Input: part model. Units: mm. Frame: model coordinates. Face numbers are marked on the shaded views. A direction names the side the tool comes from. Round coordinates to 2 decimals unless told otherwise and drop trailing zeros. Loops run counter-clockwise (first coordinate to the right, second up) from the corner with the lowest first, then second, coordinate; pieces in that order, holes last.
(1) First-contact query: pin 1 Ø1 at (x, y) = (17.5, 2) entering from +Z. Flat tip, straight axial feed; report the tip coordinate or a pass-through.
(2) Line query: line 1 (X direction, y = 2, z = 1.25); line 2 (X direction, y = 2, z = 3.1); line 3 (Y direction, x = 2.5, z = 1.85). Output: solid intervals per line, ascending.
(3) Draft query along Y for the marked faces 1, 2 and 3. Return one class per face: released by +Y, released by -Y, zero draft, split by the parting line, or undercut.
(4) Cut plane B-B, the plane z = 1.25. Output: boundary loops of the cut face in (x, y), and give its area (3 significant figures).
(5) Cut plane D-D, the plane z = 3. Output: boundary loops of the cut face in (x, y), and give its area (3 significant figures).
(6) Cut plane A-A, the plane y = 2. Output: boundary loops of the cut face in (x, z).
(7) Cut plane C-C, the plane x = 2.5. Output: boundary loops of the cut face in (y, z), and give its area (3 significant figures).
(8) Access query for the marked faces 4 and 5. Directions: +Z, -Z, +X, -X, +Y, -Y. A direction counts if a zero-diameter tool reaches every point of the face in a straight line with its end or side. Return the directions, or none.
Autodesk Inventor part; units mm, degrees
ref_plane "YZ Plane" through (0, 0, 0) normal (1, 0, 0) x (0, 1, 0)
ref_plane "XZ Plane" through (0, 0, 0) normal (0, 1, 0) x (-1, 0, 0)
ref_plane "XY Plane" through (0, 0, 0) normal (0, 0, 1) x (1, 0, 0)
sketch "Sketch1" plane through (0, 0, 0) normal (0, 0, 1) x (1, 0, 0)
  line L0 (0, 0) -> (20, 0)
  line L1 (20, 0) -> (20, 4)
  line L2 (20, 4) -> (0, 4)
  line L3 (0, 4) -> (0, 0)
  dimension "d0" = 20
  dimension "d1" = 4
extrude "Extrusion1" add sketch "Sketch1" along normal blind 4
sketch "Sketch2" plane through (0, 0, 0) normal (0, -1, 0) x (1, 0, 0)
  line L0 (5.5, 0) -> (14.5, 0)
  line L1 (14.5, 0) -> (14.5, 2)
  line L2 (14.5, 2) -> (5.5, 2)
  line L3 (5.5, 2) -> (5.5, 0)
  line L4 (0, 0) -> (20, 0) construction
  line L5 (10, 0) -> (10, 4) construction
  line L6 (0, 4) -> (20, 4) construction
  dimension "d4" = 9
  dimension "d5" = 2
extrude "Extrusion2" cut sketch "Sketch2" against normal blind 4
sketch "Sketch3" plane through (0, 0, 4) normal (0, 0, 1) x (1, 0, 0)
  line L0 (0, 2) -> (20, 2) construction
  line L1 (20, 0) -> (20, 4) construction
  line L2 (14.5, 4) -> (5.5, 4) construction
  line L3 (10, 4) -> (10, 0) construction
  line L4 (5.5, 0) -> (14.5, 0) construction
  point P0 (0, 0)
  point P1 (2.5, 2)
  point P2 (17.5, 2)
  dimension "d8" = 15
hole "Hole1" at (2.5, 2, 4) at (17.5, 2, 4) direction (0, 0, -1) diameter 1.6 end through all
properties part number "encoder_mounting_clamp"
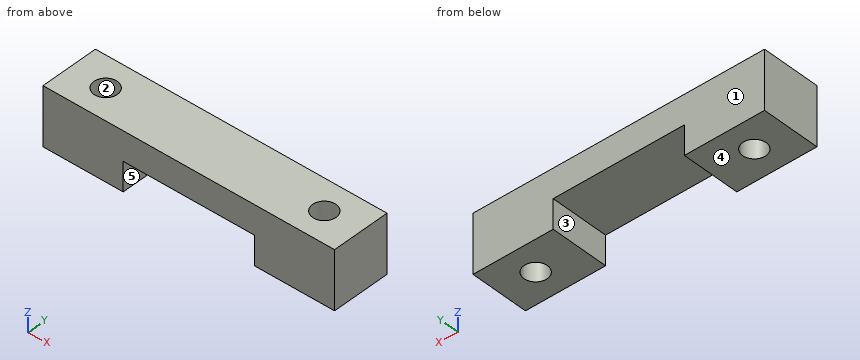
Reported:
1. pin 1: passes through
2. line 1: x = 0 to 1.7, 3.3 to 5.5, 14.5 to 16.7, 18.3 to 20
2. line 2: x = 0 to 1.7, 3.3 to 16.7, 18.3 to 20
2. line 3: y = 0 to 1.2, 2.8 to 4
3. face 1: released by +Y
3. face 2: undercut
3. face 3: zero draft
4. outline: (0, 0) - (5.5, 0) - (5.5, 4) - (0, 4) - close; (14.5, 0) - (20, 0) - (20, 4) - (14.5, 4) - close; hole circle Ø1.6 at (2.5, 2); hole circle Ø1.6 at (17.5, 2)
4. area: 40.0 mm2
5. outline: (0, 0) - (20, 0) - (20, 4) - (0, 4) - close; hole circle Ø1.6 at (2.5, 2); hole circle Ø1.6 at (17.5, 2)
5. area: 76.0 mm2
6. outline: (0, 0) - (1.7, 0) - (1.7, 4) - (0, 4) - close; (3.3, 0) - (5.5, 0) - (5.5, 2) - (14.5, 2) - (14.5, 0) - (16.7, 0) - (16.7, 4) - (3.3, 4) - close; (18.3, 0) - (20, 0) - (20, 4) - (18.3, 4) - close
7. outline: (0, 0) - (1.2, 0) - (1.2, 4) - (0, 4) - close; (2.8, 0) - (4, 0) - (4, 4) - (2.8, 4) - close
7. area: 9.60 mm2
8. face 4: -Z, +X, -X, +Y, -Y
8. face 5: -Z, +Y, -Y
